Geometry: final body of the model. Coordinates: model frame, mm. Face numbers are marked on the shaded views. A direction names the side the tool comes from. Give positions to 0.01 mm unless a question says otherwise; leave off trailing zeros. Loops run counter-clockwise (first coordinate to the right, second up) from the corner with the lowest first, then second, coordinate; pieces in that order, holes last. Notation, with made-up numbers: (-21, -15.5) -> (7, -15.5) arc R11 ccw to (7, -7.5) -> close; hole circle Ø2 at (33, -6). An arc over 180 degrees is marked (long way). One line per item, written item: value. Start each with the question number.
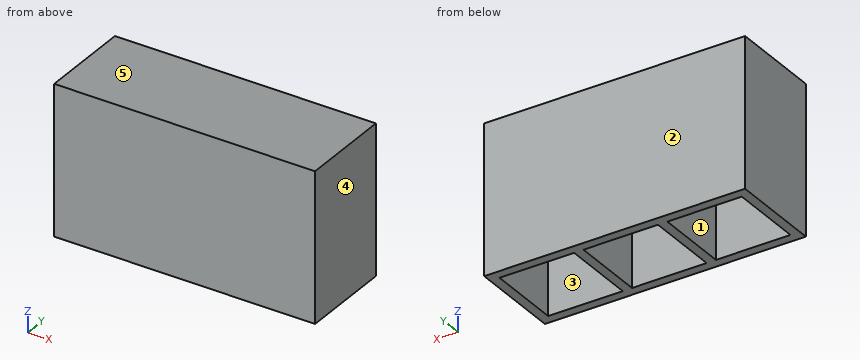
from build123d import *

# Parameters (mm, degrees)
SKETCH_1_W          = 140
SKETCH_1_H          = 50
EXTRUDE_1_DEPTH     = 80
SKETCH_3_W          = 40
SKETCH_3_H          = 40
CUT_EXTRUDE_3_DEPTH = 75


with BuildPart() as part:
    # 草图1 → 凸台-拉伸1 (new body)
    with BuildSketch(Plane.XY):
        with Locations((-29.932659933, 5.892255892)):
            Rectangle(SKETCH_1_W, SKETCH_1_H)
    extrude(amount=EXTRUDE_1_DEPTH)

    # 草图3 → 切除-拉伸3 (cut)
    with BuildSketch(Plane(origin=(0, 0, 0), x_dir=(-1, 0, 0), z_dir=(0, 0, -1))):
        with Locations((29.932659933, 5.892255892)):
            Rectangle(SKETCH_3_W, SKETCH_3_H)
        with Locations((-15.067340067, 5.892255892)):
            Rectangle(SKETCH_3_W, SKETCH_3_H)
        with Locations((74.932659933, 5.892255892)):
            Rectangle(SKETCH_3_W, SKETCH_3_H)
    extrude(amount=-CUT_EXTRUDE_3_DEPTH, mode=Mode.SUBTRACT)


solid = part.part
Item 1: Access query for the marked faces 1 and 2. Directions: +Z, -Z, +X, -X, +Y, -Y. A direction counts if a zero-diameter tool reaches every point of the face in a straight line with its end or side. Return the directions, or none.
Item 2: Section C-C, the plane y = -0.5. Output: boundary loops of the cut face in (x, z), then the cut area to 3 significant figures.
Item 3: Ray query, line 1 along X through (y, z) = (12, 63.5); line 2 along Y through (x, z) = (-32, 59); line 3 along Z through (x, y) = (-65, -11). Return the intervals inside material, ascending. Write a range as [from, to].
Item 4: Mould query, pull axis X, two halves, no side actions, for the marked faces 3, 4 and 5. Classes: pulls with the +X half, pulls with the -X half, needs draft (parallel to the pull), parting line crosses it, or undercut.
Item 5: Section B-B, the plane x = 20. Output: boundary loops of the cut face in (y, z).
Item 6: Section A-A, the plane z = 25.5. Output: boundary loops of the cut face in (x, y), then the cut area to 3 significant figures.
Item 7: Pin query (flat end, axial travel): pin 1 (20 mm diameter, centred on x = -28.5, y = 3.5, fed in from -Z). Return the tip coordinate at first contact, or that it passes through.
Geometry check:
1. face 1: -Z
1. face 2: +Z, -Z, +X, -X, +Y
2. outline: (-99.93, 0) -> (-94.93, 0) -> (-94.93, 75) -> (-54.93, 75) -> (-54.93, 0) -> (-49.93, 0) -> (-49.93, 75) -> (-9.93, 75) -> (-9.93, 0) -> (-4.93, 0) -> (-4.93, 75) -> (35.07, 75) -> (35.07, 0) -> (40.07, 0) -> (40.07, 80) -> (-99.93, 80) -> close
2. area: 2,200 mm2
3. line 1: x = [-99.93, -94.93], [-54.93, -49.93], [-9.93, -4.93], [35.07, 40.07]
3. line 2: y = [-19.11, -14.11], [25.89, 30.89]
3. line 3: z = [75, 80]
4. face 3: undercut
4. face 4: pulls with the +X half
4. face 5: needs draft
5. outline: (-19.11, 0) -> (-14.11, 0) -> (-14.11, 75) -> (25.89, 75) -> (25.89, 0) -> (30.89, 0) -> (30.89, 80) -> (-19.11, 80) -> close
6. outline: (-99.93, -19.11) -> (40.07, -19.11) -> (40.07, 30.89) -> (-99.93, 30.89) -> close; hole (-94.93, -14.11) -> (-54.93, -14.11) -> (-54.93, 25.89) -> (-94.93, 25.89) -> close; hole (-49.93, -14.11) -> (-9.93, -14.11) -> (-9.93, 25.89) -> (-49.93, 25.89) -> close; hole (-4.93, -14.11) -> (35.07, -14.11) -> (35.07, 25.89) -> (-4.93, 25.89) -> close
6. area: 2,200 mm2
7. pin 1: stops at z = 75
